```python
from build123d import *

# Parameters (mm, degrees)
CYLINDER222_R     = 1.25
CYLINDER222_DEPTH = 22
CYLINDER221_R     = 4.65
CYLINDER221_DEPTH = 13
BOX148_W          = 20
BOX148_H          = 20
BOX148_DEPTH      = 3
CHAMFER007_SIZE   = 2
BOX149_W          = 16
BOX149_H          = 3.5
BOX149_DEPTH      = 8.5
CHAMFER008_SIZE   = 6.5
BOX147_W          = 16
BOX147_H          = 3.5
BOX147_DEPTH      = 8.5
CHAMFER006_SIZE   = 6.5
FILLET064_R       = 3
FILLET063_R       = 2.49
FILLET062_R       = 0.5


with BuildPart() as cylinder494:
    # Cylinder222 → Cylinder222 (new body)
    with BuildSketch(Plane(origin=(320, 13, -68), x_dir=(1, 0, 0), z_dir=(0, -1, 0))):
        Circle(CYLINDER222_R)
    extrude(amount=CYLINDER222_DEPTH)


with BuildPart() as cylinder493:
    # Cylinder221 → Cylinder221 (new body)
    with BuildSketch(Plane(origin=(320, -4.5, -68), x_dir=(1, 0, 0), z_dir=(0, 1, 0))):
        Circle(CYLINDER221_R)
    extrude(amount=CYLINDER221_DEPTH)


with BuildPart() as chamfer007:
    # Box148 → Box148 (new body)
    with BuildSketch(Plane(origin=(310, -8, -74), x_dir=(1, 0, 0), z_dir=(0, 0, 1))):
        with Locations((10, 10)):
            Rectangle(BOX148_W, BOX148_H)
    extrude(amount=BOX148_DEPTH)

    # Cut156: cut Cylinder493
    add(cylinder493.part, mode=Mode.SUBTRACT)

    # Chamfer007
    chamfer007_edges = [chamfer007.edges().sort_by_distance(p)[0] for p in [
        (323.552816, 2, -71),
        (316.447184, 2, -71),
    ]]
    chamfer(chamfer007_edges, length=CHAMFER007_SIZE)


with BuildPart() as chamfer008:
    # Box149 → Box149 (new body)
    with BuildSketch(Plane(origin=(311, 8.5, -74), x_dir=(1, 0, 0), z_dir=(0, 0, 1))):
        with Locations((8, 1.75)):
            Rectangle(BOX149_W, BOX149_H)
    extrude(amount=BOX149_DEPTH)

    # Chamfer008
    chamfer008_edges = [chamfer008.edges().sort_by_distance(p)[0] for p in [
        (311, 10.25, -65.5),
        (327, 10.25, -65.5),
    ]]
    chamfer(chamfer008_edges, length=CHAMFER008_SIZE)


with BuildPart() as chamfer008_1:
    # Chamfer008 placement: moved
    add(chamfer008.part.moved(Location((1, 0, 0))))


with BuildPart() as supports_right_foot:
    # Box147 → Box147 (new body)
    with BuildSketch(Plane(origin=(311, 8.5, -74), x_dir=(1, 0, 0), z_dir=(0, 0, 1))):
        with Locations((8, 1.75)):
            Rectangle(BOX147_W, BOX147_H)
    extrude(amount=BOX147_DEPTH)

    # Chamfer006
    chamfer006_edges = [supports_right_foot.edges().sort_by_distance(p)[0] for p in [
        (311, 10.25, -65.5),
        (327, 10.25, -65.5),
    ]]
    chamfer(chamfer006_edges, length=CHAMFER006_SIZE)


with BuildPart() as supports_right_foot_1:
    # Chamfer006 placement: moved
    add(supports_right_foot.part.moved(Location((1, -16.5, 0))))

    # Fusion190: union Chamfer007, Chamfer008
    add(chamfer007.part)
    add(chamfer008_1.part)

    # Fillet064
    fillet064_edges = [supports_right_foot_1.edges().sort_by_distance(p)[0] for p in [
        (318.5, -6.25, -65.5),
        (321.5, -6.25, -65.5),
        (318.5, 10.25, -65.5),
        (321.5, 10.25, -65.5),
    ]]
    fillet(fillet064_edges, radius=FILLET064_R)

    # Fillet063
    fillet063_edges = [supports_right_foot_1.edges().sort_by_distance(p)[0] for p in [
        (330, 2, -74),
        (310, 2, -74),
    ]]
    fillet(fillet063_edges, radius=FILLET063_R)

    # Fillet062
    fillet062_edges = [supports_right_foot_1.edges().sort_by_distance(p)[0] for p in [
        (330, 2, -71),
        (310, 2, -71),
    ]]
    fillet(fillet062_edges, radius=FILLET062_R)

    # Cut155: cut Cylinder494
    add(cylinder494.part, mode=Mode.SUBTRACT)


with BuildPart() as supports_right_foot_2:
    # Cut155 placement: moved
    add(supports_right_foot_1.part.moved(Location((-77.3, 77, 16))))


solid = supports_right_foot_2.part
```
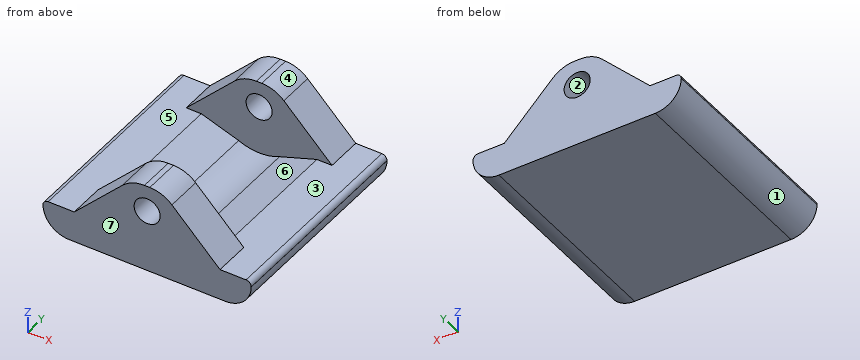
Verification items for the finished model (mm, model axes). Face numbers are marked on the shaded views. A direction names the side the tool comes from. Coordinates: 2 decimals unless noted, no trailing zeros. Loops run counter-clockwise (first coordinate to the right, second up) from the corner with the lowest first, then second, coordinate; pieces in that order, holes last. Notation, with made-up numbers: (43, -26) - (87, -26) arc R15 cw to (87, 1) - close; hole circle Ø10 at (25.5, 48.5). An arc over 180 degrees is marked (long way). Answer as a JSON object with one key per item and string values.
(1) Scan lines: line 1 along Y through (x, z) = (244.25, -53.75); line 2 along Z through (x, y) = (242.7, 71.7); line 3 along X through (y, z) = (86.85, -52). Record each from-to range of solid material in increasing order.
Response:
{"line 1": "y = 69 to 72.5, 85.5 to 89", "line 2": "z = -58 to -53.25, -50.75 to -49.5", "line 3": "x = 238.7 to 241.45, 243.95 to 246.7"}
(2) Cross-section at B-B, the plane z = -51.25. Record the boundary of the cut face in (x, y), then the cut area to 3 significant figures.
Response:
{"outline": "(239.45, 69) - (241.7, 69) - (241.7, 72.5) - (239.45, 72.5) - close; (239.45, 85.5) - (241.7, 85.5) - (241.7, 89) - (239.45, 89) - close; (243.7, 69) - (245.95, 69) - (245.95, 72.5) - (243.7, 72.5) - close; (243.7, 85.5) - (245.95, 85.5) - (245.95, 89) - (243.7, 89) - close", "area": "31.5 mm²"}
(3) Cross-section at C-C, the plane z = -53.75. Record the boundary of the cut face in (x, y).
Response:
{"outline": "(236.95, 69) - (248.45, 69) - (248.45, 72.5) - (236.95, 72.5) - close; (236.95, 85.5) - (248.45, 85.5) - (248.45, 89) - (236.95, 89) - close"}
(4) Go/stop test with flat-tipped pins: pin 1 Ø3 at (x, z) = (242.7, -52) entering from +Y; pin 2 Ø3 at (x, y) = (249.5, 80.5) entering from +Z. Record where each tip stops, or that it passes through.
Response:
{"pin 1": "stops at y = 89", "pin 2": "stops at z = -55"}
(5) Access from +Z, -Z, +X, -X, +Y, -Y to the whole of each face (thin tool, end or side, straight path). Record for the marked faces 5, 6 and 7.
Response:
{"face 5": "+Z, -X", "face 6": "+Z", "face 7": "+Z, -Z, +X, -X, -Y"}
(6) Cross-section at A-A, the plane x = 242.7. Record the boundary of the cut face in (y, z).
Response:
{"outline": "(69, -58) - (89, -58) - (89, -53.25) - (85.5, -53.25) - (85.5, -56.65) - (72.5, -56.65) - (72.5, -53.25) - (69, -53.25) - close; (69, -50.75) - (72.5, -50.75) - (72.5, -49.5) - (69, -49.5) - close; (85.5, -50.75) - (89, -50.75) - (89, -49.5) - (85.5, -49.5) - close"}
(7) Mould release check, pull along X, two halves, no side actions. Record for the marked faces 1, 2, 3 and 4: pulls with the +X half, pulls with the -X half, needs draft (parallel to the pull), parting line crosses it, or undercut.
Response:
{"face 1": "pulls with the -X half", "face 2": "undercut", "face 3": "needs draft", "face 4": "pulls with the +X half"}
